from build123d import *

# Parameters (mm, degrees)
F0_R     = 40
F0_R_2   = 15
F1_DEPTH = 5
F0_R_3   = 8.5
F2_DEPTH = 4
F0_R_4   = 7.5
F3_DEPTH = 5
F0_R_5   = 4.05
F4_DEPTH = 1


with BuildPart() as f1:
    # F0 (on Top) → F1 (new body)
    with BuildSketch(Plane.XY):
        Circle(F0_R)
        with BuildLine():
            ThreePointArc((-11.961144, -30.637533), (-19.071879, -33.033464), (-20.55231, -25.677421))
            Line((-20.55231, -25.677421), (-13.40868, -16.280358))
            ThreePointArc((-13.40868, -16.280358), (-8.872378, -15.36741), (-7.394863, -19.752436))
            Line((-7.394863, -19.752436), (-11.961144, -30.637533))
        make_face(mode=Mode.SUBTRACT)
        with BuildLine():
            ThreePointArc((4.960112, -32.513454), (0, -38.143759), (-4.960112, -32.513454))
            Line((-4.960112, -32.513454), (-3.472079, -20.803543))
            ThreePointArc((-3.472079, -20.803543), (0, -17.744757), (3.472079, -20.803543))
            Line((3.472079, -20.803543), (4.960112, -32.513454))
        make_face(mode=Mode.SUBTRACT)
        with BuildLine():
            ThreePointArc((-25.677421, -20.55231), (-33.033464, -19.071879), (-30.637533, -11.961144))
            Line((-30.637533, -11.961144), (-19.752436, -7.394863))
            ThreePointArc((-19.752436, -7.394863), (-15.36741, -8.872378), (-16.280358, -13.40868))
            Line((-16.280358, -13.40868), (-25.677421, -20.55231))
        make_face(mode=Mode.SUBTRACT)
        with BuildLine():
            ThreePointArc((20.55231, -25.677421), (19.071879, -33.033464), (11.961144, -30.637533))
            Line((11.961144, -30.637533), (7.394863, -19.752436))
            ThreePointArc((7.394863, -19.752436), (8.872378, -15.36741), (13.40868, -16.280358))
            Line((13.40868, -16.280358), (20.55231, -25.677421))
        make_face(mode=Mode.SUBTRACT)
        with BuildLine():
            ThreePointArc((30.637533, -11.961144), (33.033464, -19.071879), (25.677421, -20.55231))
            Line((25.677421, -20.55231), (16.280358, -13.40868))
            ThreePointArc((16.280358, -13.40868), (15.36741, -8.872378), (19.752436, -7.394863))
            Line((19.752436, -7.394863), (30.637533, -11.961144))
        make_face(mode=Mode.SUBTRACT)
        with BuildLine():
            ThreePointArc((32.513454, 4.960112), (38.143759, 0), (32.513454, -4.960112))
            Line((32.513454, -4.960112), (20.803543, -3.472079))
            ThreePointArc((20.803543, -3.472079), (17.744757, 0), (20.803543, 3.472079))
            Line((20.803543, 3.472079), (32.513454, 4.960112))
        make_face(mode=Mode.SUBTRACT)
        with BuildLine():
            ThreePointArc((-32.513454, -4.960112), (-38.143759, 0), (-32.513454, 4.960112))
            Line((-32.513454, 4.960112), (-20.803543, 3.472079))
            ThreePointArc((-20.803543, 3.472079), (-17.744757, 0), (-20.803543, -3.472079))
            Line((-20.803543, -3.472079), (-32.513454, -4.960112))
        make_face(mode=Mode.SUBTRACT)
        with BuildLine():
            ThreePointArc((-30.637533, 11.961144), (-33.033464, 19.071879), (-25.677421, 20.55231))
            Line((-25.677421, 20.55231), (-16.280358, 13.40868))
            ThreePointArc((-16.280358, 13.40868), (-15.36741, 8.872378), (-19.752436, 7.394863))
            Line((-19.752436, 7.394863), (-30.637533, 11.961144))
        make_face(mode=Mode.SUBTRACT)
        with BuildLine():
            ThreePointArc((-20.55231, 25.677421), (-19.071879, 33.033464), (-11.961144, 30.637533))
            Line((-11.961144, 30.637533), (-7.394863, 19.752436))
            ThreePointArc((-7.394863, 19.752436), (-8.872378, 15.36741), (-13.40868, 16.280358))
            Line((-13.40868, 16.280358), (-20.55231, 25.677421))
        make_face(mode=Mode.SUBTRACT)
        Circle(F0_R_2, mode=Mode.SUBTRACT)
        with BuildLine():
            ThreePointArc((25.677421, 20.55231), (33.033464, 19.071879), (30.637533, 11.961144))
            Line((30.637533, 11.961144), (19.752436, 7.394863))
            ThreePointArc((19.752436, 7.394863), (15.36741, 8.872378), (16.280358, 13.40868))
            Line((16.280358, 13.40868), (25.677421, 20.55231))
        make_face(mode=Mode.SUBTRACT)
        with BuildLine():
            ThreePointArc((3.472079, 20.803543), (0, 17.744757), (-3.472079, 20.803543))
            Line((-3.472079, 20.803543), (-4.960112, 32.513454))
            ThreePointArc((-4.960112, 32.513454), (0, 38.143759), (4.960112, 32.513454))
            Line((4.960112, 32.513454), (3.472079, 20.803543))
        make_face(mode=Mode.SUBTRACT)
        with BuildLine():
            ThreePointArc((11.961144, 30.637533), (19.071879, 33.033464), (20.55231, 25.677421))
            Line((20.55231, 25.677421), (13.40868, 16.280358))
            ThreePointArc((13.40868, 16.280358), (8.872378, 15.36741), (7.394863, 19.752436))
            Line((7.394863, 19.752436), (11.961144, 30.637533))
        make_face(mode=Mode.SUBTRACT)
    extrude(amount=F1_DEPTH)

    # F0 (on Top) → F2 (join)
    with BuildSketch(Plane.XY):
        Circle(F0_R_2)
        Circle(F0_R_3, mode=Mode.SUBTRACT)
    extrude(amount=F2_DEPTH)

    # F0 (on Top) → F3 (join)
    with BuildSketch(Plane.XY):
        Circle(F0_R_3)
        Circle(F0_R_4, mode=Mode.SUBTRACT)
    extrude(amount=F3_DEPTH)

    # F0 (on Top) → F4 (join)
    with BuildSketch(Plane.XY):
        Circle(F0_R_4)
        Circle(F0_R_5, mode=Mode.SUBTRACT)
    extrude(amount=F4_DEPTH)


solid = f1.part
Check sheet for the modelled part. Datum: model origin and axes. Units: mm. A direction names the side the tool comes from. Coordinates: 2 decimals unless noted, no trailing zeros. Write each loop counter-clockwise with the first axis right and the second up, starting at its lowest first coordinate (ties: lowest second). Pieces come first, ordered by that corner, then holes. Notation, with made-up numbers: M 48.5,27.25 L 72.5,27.25 A24 cw 72.5,57.25 Z; hole C 16.25,41.5 d2. An arc over 180 degrees is marked long. Answer as CSV lines item,"result".
Q1. Mould release check, pull along Y, two halves, no side actions. Record for faces 1 (the face through (0, -8, 5)), 2 (the face through (-25.119, 9.646, 2.465)): released by +Y, released by -Y, zero draft, split by the parting line, or undercut.
Check result:
face 1,"zero draft"
face 2,"undercut"
Q2. Cross-section at D-D (z = 2.25). Count the separate pieces of the cut face and the enclosed holes in it, then the cut area to 3 significant figures.
Check result:
separate pieces,"1"
enclosed holes,"13"
area,"2,920 mm^2"
Q3. Set-up check for faces 3 (the face through (8, 1, 0)), 4 (the face through (25.27, 9.71, 2.46)), 5 (the face through (3, -3, 1)): record each of +Z, -Z, +X, -X, +Y, -Y from which the full face is reachable in a straight line by a thin tool's end or side.
Check result:
face 3,"-Z, +X, -X, +Y, -Y"
face 4,"+Z, -Z"
face 5,"+Z"
Q4. Cross-section at C-C (x = 11). Record the boundary of the cut face in (y, z), then the cut area to 3 significant figures.
Check result:
outline,"M -38.46,0 L -28.35,0 L -28.35,5 L -38.46,5 Z; M -14.92,0 L 14.92,0 L 14.92,5 L 10.2,5 L 10.2,4 L -10.2,4 L -10.2,5 L -14.92,5 Z; M 28.35,0 L 38.46,0 L 38.46,5 L 28.35,5 Z"
area,"230 mm^2"
Q5. Cross-section at A-A (x = 0). Record the boundary of the cut face in (y, z), then the cut area to 3 significant figures.
Check result:
outline,"M -40,0 L -38.14,0 L -38.14,5 L -40,5 Z; M -17.74,0 L -4.05,0 L -4.05,1 L -7.5,1 L -7.5,5 L -8.5,5 L -8.5,4 L -15,4 L -15,5 L -17.74,5 Z; M 4.05,0 L 17.74,0 L 17.74,5 L 15,5 L 15,4 L 8.5,4 L 8.5,5 L 7.5,5 L 7.5,1 L 4.05,1 Z; M 38.14,0 L 40,0 L 40,5 L 38.14,5 Z"
area,"115 mm^2"
Q6. Go/stop test with flat-tipped pins: pin 1 (6 mm diameter, centred on x = 16.57, y = 28.7, fed in from +Z); pin 2 (3 mm diameter, centred on y = 22, z = 2.5, fed in from +X); pin 3 (9 mm diameter, centred on x = 0, y = 0, fed in from +Z); pin 4 (1 mm diameter, centred on y = 18, z = 2.5, fed in from -X). Record where each tip stops, or that it passes through.
Check result:
pin 1,"through"
pin 2,"x = 34.35"
pin 3,"z = 1"
pin 4,"x = -35.97"
Q7. Material ranges on probe 1 along X at (y, z) = (25, 2.25); probe 2 along X at (y, z) = (33, 3); probe 3 along Y at (x, z) = (-28.5, 4.4), recorded low to high. Write a range as from..to.
Check result:
probe 1,"-31.22..-20.04, -9.6..-4.01, 4.01..9.6, 20.04..31.22"
probe 2,"-22.61..-19.13, -14.01..-5, 5..14.01, 19.13..22.61"
probe 3,"-28.07..-21.57, -11.06..-4.45, 4.45..11.06, 21.57..28.07"
